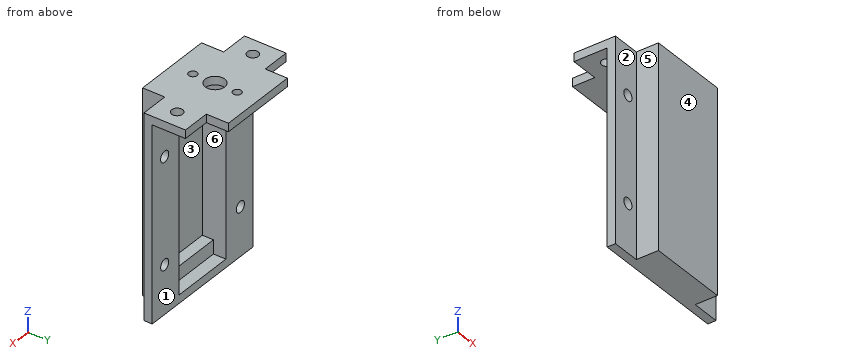
from build123d import *

# Parameters (mm, degrees)
SALIENTE_EXTRUIR2_DEPTH = 3
SALIENTE_EXTRUIR3_DEPTH = 70
CROQUIS_HUECO_MOTOR_W   = 23
CROQUIS_HUECO_MOTOR_H   = 67
HUECO_MOTOR_DEPTH       = 8.5
CROQUIS10_R             = 3.5
CROQUIS10_R_2           = 2
CROQUIS10_R_3           = 1.5
TORNILLO_Y_MOTOR_DEPTH  = 5
CROQUIS12_W             = 23
CROQUIS12_H             = 5
SALIENTE_EXTRUIR5_DEPTH = 4
CROQUIS16_R             = 2
CORTAR_EXTRUIR4_DEPTH   = 77.893188905


with BuildPart() as part:
    # Croquis4 → Saliente-Extruir2 (new body)
    with BuildSketch(Plane.XY):
        Polygon((14.5, 16), (-14.5, 16), (-14.5, 8), (-24.75, 8), (-24.75, -7), (-14.5, -7), (-14.5, -15), (14.5, -15), (14.5, -7), (24.75, -7), (24.75, 8), (14.5, 8), align=None)
    extrude(amount=SALIENTE_EXTRUIR2_DEPTH)

    # Croquis5 → Saliente-Extruir3 (add)
    with BuildSketch(Plane(origin=(0, 0, 0), x_dir=(-1, 0, 0), z_dir=(0, 0, -1))):
        Polygon((-24.75, -4), (-24.75, -7), (-14.5, -7), (-14.5, -15), (14.5, -15), (14.5, -7), (24.75, -7), (24.75, -4), align=None)
    extrude(amount=SALIENTE_EXTRUIR3_DEPTH)

    # croquis hueco motor → hueco motor (cut)
    with BuildSketch(Plane(origin=(0, -4, 0), x_dir=(1, 0, 0), z_dir=(0, 1, 0))):
        with Locations((0, 33.5)):
            Rectangle(CROQUIS_HUECO_MOTOR_W, CROQUIS_HUECO_MOTOR_H)
    extrude(amount=-HUECO_MOTOR_DEPTH, mode=Mode.SUBTRACT)

    # Croquis10 → tornillo y motor (cut)
    with BuildSketch(Plane.XY.offset(3)):
        with Locations((0, 0.5)):
            Circle(CROQUIS10_R)
        with Locations((-18.6, 0.5)):
            Circle(CROQUIS10_R_2)
        with Locations(Location((18.6, 0.5, 0), (0, 0, 180))):
            Circle(CROQUIS10_R_2)
        with Locations((0, 8.5)):
            Circle(CROQUIS10_R_3)
        with Locations(Location((0, -7.5, 0), (0, 0, 180))):
            Circle(CROQUIS10_R_3)
    extrude(amount=-TORNILLO_Y_MOTOR_DEPTH, mode=Mode.SUBTRACT)

    # Croquis12 → Saliente-Extruir5 (add)
    with BuildSketch(Plane(origin=(0, -12.5, 0), x_dir=(1, 0, 0), z_dir=(0, 1, 0))):
        with Locations((0, 64.5)):
            Rectangle(CROQUIS12_W, CROQUIS12_H)
    extrude(amount=SALIENTE_EXTRUIR5_DEPTH)

    # Croquis16 → Cortar-Extruir4 (cut, through all)
    with BuildSketch(Plane(origin=(0, -4, 0), x_dir=(1, 0, 0), z_dir=(0, 1, 0))):
        with Locations(Location((-18.63, 52.5, 0), (0, 0, 180))):
            Circle(CROQUIS16_R)
        with Locations(Location((-18.63, 14.5, 0), (0, 0, 270))):
            Circle(CROQUIS16_R)
        with Locations(Location((18.63, 14.5, 0), (0, 0, 180))):
            Circle(CROQUIS16_R)
        with Locations(Location((18.63, 52.5, 0), (0, 0, 180))):
            Circle(CROQUIS16_R)
    extrude(amount=-CORTAR_EXTRUIR4_DEPTH, mode=Mode.SUBTRACT)


solid = part.part
CAD build for the part. Positions are in the model's coordinates, mm. Face numbers are marked on the shaded views. A direction names the side the tool comes from. Coordinates: 2 decimals unless noted, no trailing zeros. Order: outer loops, then holes, each group sorted by start corner. A loop starts at its lowest first (then second) coordinate and runs counter-clockwise, first axis right, second up. Notation, with made-up numbers: (-13, -30.5) -> (11, -30.5) arc R32 ccw to (11, 4.5) -> close; hole circle Ø3 at (76, 78). An arc over 180 degrees is marked (long way). Answer in a Markdown table with one row per item.
1) Band-saw the part on A-A (y = 0.5). List the corners of the cut face in (x, z).
Check values:
| item | result |
|---|---|
| outline | (-24.75, 0) -> (-20.6, 0) -> (-20.6, 3) -> (-24.75, 3) -> close; (-16.6, 0) -> (-3.5, 0) -> (-3.5, 3) -> (-16.6, 3) -> close; (3.5, 0) -> (16.6, 0) -> (16.6, 3) -> (3.5, 3) -> close; (20.6, 0) -> (24.75, 0) -> (24.75, 3) -> (20.6, 3) -> close |
2) Band-saw the part on B-B (z = -41). List the corners of the cut face in (x, y).
Check values:
| item | result |
|---|---|
| outline | (-24.75, -7) -> (-14.5, -7) -> (-14.5, -15) -> (14.5, -15) -> (14.5, -7) -> (24.75, -7) -> (24.75, -4) -> (11.5, -4) -> (11.5, -12.5) -> (-11.5, -12.5) -> (-11.5, -4) -> (-24.75, -4) -> close |
3) Flat gauge pins, fed straight in: P1, Ø8, axis at x = 20.5, z = -39.5, coming from the -Y side; P2, Ø8, axis at x = 0, y = 0.5, coming from the -Z side; P3, Ø4.5, axis at x = -18.6, y = 0.5, coming from the +Z side; P4, Ø2.5, axis at x = 18, z = 1.5, coming from the +Y side. Where does each tip first touch, or does it go through?
Check values:
| item | result |
|---|---|
| P1 | y = -7 |
| P2 | z = 0 |
| P3 | z = 3 |
| P4 | y = 8 |
4) Band-saw the part on D-D (z = -51.5). List the corners of the cut face in (x, y), and give its area (3 significant figures).
Check values:
| item | result |
|---|---|
| outline | (-24.75, -7) -> (-20.36, -7) -> (-20.36, -4) -> (-24.75, -4) -> close; (-16.9, -7) -> (-14.5, -7) -> (-14.5, -15) -> (14.5, -15) -> (14.5, -7) -> (16.9, -7) -> (16.9, -4) -> (11.5, -4) -> (11.5, -12.5) -> (-11.5, -12.5) -> (-11.5, -4) -> (-16.9, -4) -> close; (20.36, -7) -> (24.75, -7) -> (24.75, -4) -> (20.36, -4) -> close |
| area | 164 mm2 |
5) Drill centre lines: line 1 (Y direction, x = 0, z = 1.9); line 2 (Z direction, x = -5.5, y = -12); line 3 (Z direction, x = 3.5, y = -8). Where is each one in solid material? Low to high.
Check values:
| item | result |
|---|---|
| line 1 | -15 to -9, -6 to -3, 4 to 7, 10 to 16 |
| line 2 | -70 to -62, 0 to 3 |
| line 3 | -70 to -67, 0 to 3 |
6) Band-saw the part on C-C (x = 18.6). List the corners of the cut face in (y, z).
Check values:
| item | result |
|---|---|
| outline | (-7, -70) -> (-4, -70) -> (-4, -54.5) -> (-7, -54.5) -> close; (-7, -50.5) -> (-4, -50.5) -> (-4, -16.5) -> (-7, -16.5) -> close; (-7, -12.5) -> (-4, -12.5) -> (-4, 0) -> (-1.5, 0) -> (-1.5, 3) -> (-7, 3) -> close; (2.5, 0) -> (8, 0) -> (8, 3) -> (2.5, 3) -> close |
7) Which spindle directions (+Z, -Z, +X, -X, +Y, -Y) get a long thin tool onto all of the face, cutting with end or side? Do the marked faces 1, 2 and 3. Say none if no direction does.
Check values:
| item | result |
|---|---|
| face 1 | -Z, +X, -X, +Y |
| face 2 | +Z, -Z, -X, -Y |
| face 3 | +Y |
8) Mould opens along X. For the marked faces 4, 5 and 6 say: pulls with the +X half, pulls with the -X half, needs draft (parallel to the pull), parting line crosses it, or undercut.
Check values:
| item | result |
|---|---|
| face 4 | needs draft |
| face 5 | pulls with the -X half |
| face 6 | undercut |
